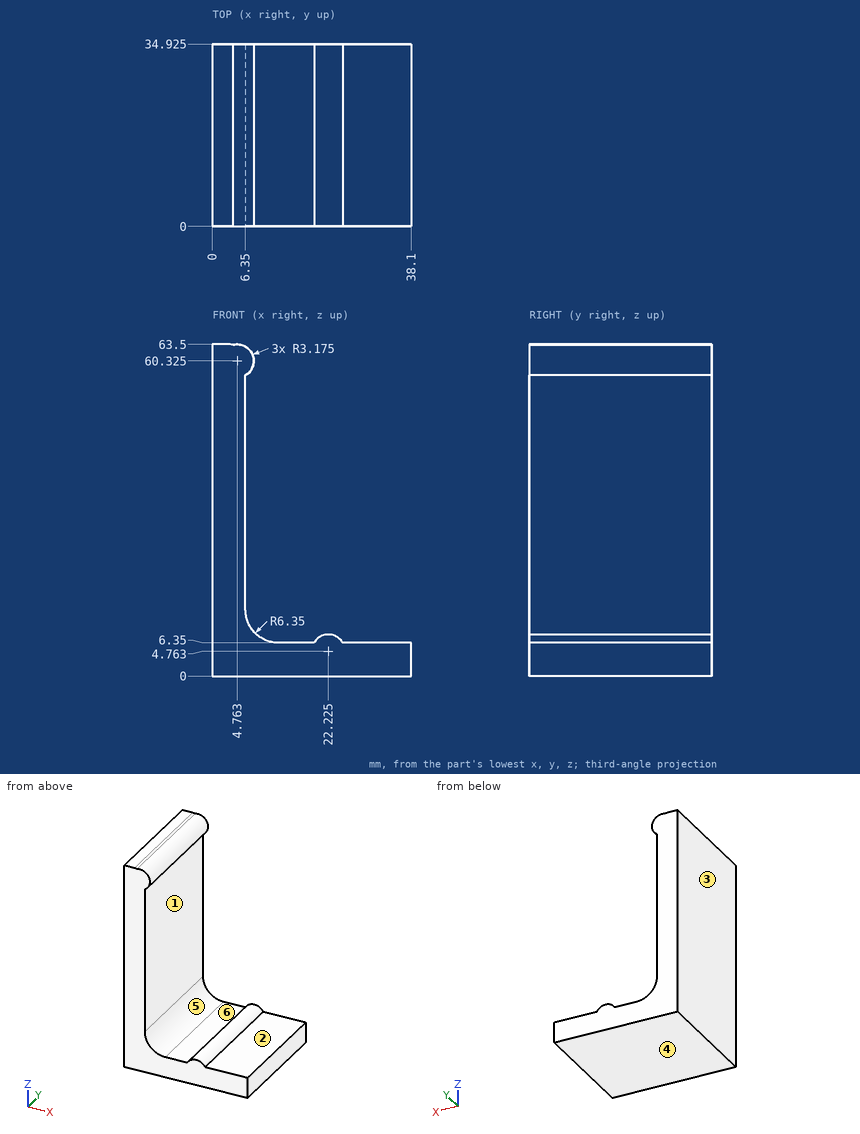
Design review of the part shown in the three views and the two pictorial views. Dimensions are in mm from the part's minimum x, y and z. A direction names the side the tool comes from. Round coordinates to 2 decimals unless told otherwise and drop trailing zeros. Write item = value, one per line. Start each with the question number.
1) Clearance check with flat-ended pins moving along their axes: pin 1 (10 mm diameter, centred on x = 12, y = 4.5, fed in from +Z); pin 2 (6.5 mm diameter, centred on x = 31.5, y = 12, fed in from +Z); pin 3 (3.5 mm diameter, centred on x = 17.5, y = 9.5, fed in from +Z). State where each tip first meets the part, or that it passes through.
2) Mouldability with a two-part tool opening along Z and no side actions: class the marked faces 4, 5 and 6 as +Z half, -Z half, draft (parallel to the pull), parting line (faces both ways), or undercut.
3) Wall thickness on probe 1 along X at (y, z) = (21, 51): over which ranges is the line inside the solid? List them lowest first. Write a range as from..to.
4) Tool access review of the marked faces 1, 2 and 3: name each direction out of +Z, -Z, +X, -X, +Y, -Y from which nothing blocks a thin tool from reaching the whole face with its end or side.
Results list:
q1.pin_1 = 62.58
q1.pin_2 = 6.35
q1.pin_3 = 6.35
q2.face_4 = -Z half
q2.face_5 = undercut
q2.face_6 = +Z half
q3.probe_1 = 0..6.35
q4.face_1 = +X, +Y, -Y
q4.face_2 = +Z, +X, +Y, -Y
q4.face_3 = +Z, -Z, -X, +Y, -Y
